CAD build for the part. Positions are in the model's coordinates, mm. Face numbers are marked on the shaded views. A direction names the side the tool comes from. Coordinates: 2 decimals unless noted, no trailing zeros. Order: outer loops, then holes, each group sorted by start corner. A loop starts at its lowest first (then second) coordinate and runs counter-clockwise, first axis right, second up. Notation, with made-up numbers: (42.5, -20.5) - (47.5, -20.5) arc R34 ccw to (47.5, 11.5) - close; hole circle Ø2 at (41, 19). An arc over 180 degrees is marked (long way). Use one line per item in the form item = value.
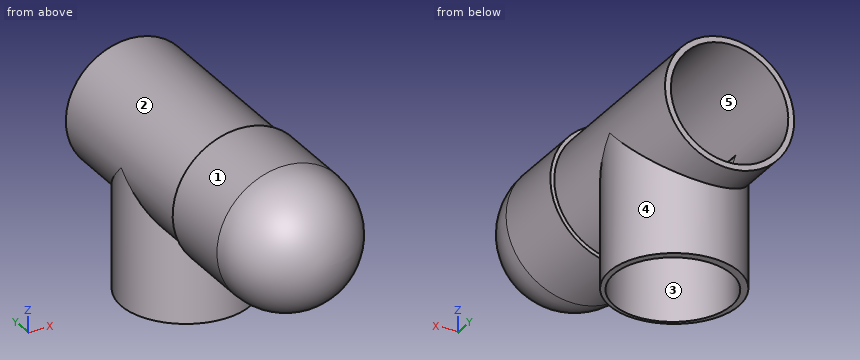
```python
from build123d import *

# Parameters (mm, degrees)
SKETCH1_R                = 15
BOSS_EXTRUDE1_DEPTH      = 70
SKETCH7_R                = 17.5
BOSS_EXTRUDE2_DEPTH      = 20
SKETCH8_R                = 16.5
SKETCH8_R_2              = 15
BOSS_EXTRUDE4_DEPTH      = 70
SKETCH10_R               = 15
CUT_EXTRUDE2_DEPTH       = 70
SKETCH24_R               = 15
CUT_EXTRUDE4_DEPTH       = 22
BOSS_EXTRUDE5_DEPTH      = 15
BOSS_EXTRUDE5_DEPTH_BACK = 20
SKETCH30_R               = 16.5
SKETCH31_R               = 15
CUT_EXTRUDE5_DEPTH       = 37
SKETCH32_R               = 15
CUT_EXTRUDE6_DEPTH       = 55


# Read off the part's stored shape, not the designer's step: Revolve1
with BuildPart() as part:
    # Sketch1 → Boss-Extrude1 (new body)
    with BuildSketch(Plane(origin=(0, 0, 0), x_dir=(1, 0, 0), z_dir=(0, 1, 0))):
        with Locations(Location((0, 0, 0), (0, 0, 270))):
            Circle(SKETCH1_R)
    extrude(amount=-BOSS_EXTRUDE1_DEPTH)

    # Sketch7 → Boss-Extrude2 (add)
    with BuildSketch(Plane.XZ.offset(70)):
        with Locations(Location((0, 0, 0), (0, 0, 270))):
            Circle(SKETCH7_R)
    extrude(amount=-BOSS_EXTRUDE2_DEPTH)

    # Sketch8 → Boss-Extrude4 (add)
    with BuildSketch(Plane(origin=(0, 0, 0), x_dir=(1, 0, 0), z_dir=(0, 1, 0))):
        with Locations(Location((0, 0, 0), (0, 0, 270))):
            Circle(SKETCH8_R)
        Circle(SKETCH8_R_2, mode=Mode.SUBTRACT)
    extrude(amount=-BOSS_EXTRUDE4_DEPTH)

    # Sketch10 → Cut-Extrude2 (cut)
    with BuildSketch(Plane(origin=(0, 0, 0), x_dir=(1, 0, 0), z_dir=(0, 1, 0))):
        with Locations(Location((0, 0, 0), (0, 0, 270))):
            Circle(SKETCH10_R)
    extrude(amount=-CUT_EXTRUDE2_DEPTH, mode=Mode.SUBTRACT)

    # Revolve1 outline → Revolve1 (revolve)
    with BuildSketch(Plane.XY):
        with BuildLine():
            Line((17.5, -69.999999983), (0, -69.999999992))
            Line((0, -69.999999992), (0, -87.5))
            ThreePointArc((0, -87.5), (12.374368677, -82.374368665), (17.5, -69.999999983))
        make_face()
    revolve(axis=Axis((0, 0, 0), (0, 1, 0)))

    # Sketch24 → Cut-Extrude4 (cut)
    with BuildSketch(Plane.XY):
        with Locations((0, -25)):
            Circle(SKETCH24_R)
    extrude(amount=-CUT_EXTRUDE4_DEPTH, mode=Mode.SUBTRACT)

    # Sketch28 → Cut-Revolve1 (revolve, cut)
    with BuildSketch(Plane.XY):
        with BuildLine():
            Line((15, -70), (-15, -70))
            ThreePointArc((-15, -70), (0, -85), (15, -70))
        make_face()
    revolve(axis=Axis((-15, -70, 0), (1, 0, 0)), mode=Mode.SUBTRACT)

    # Sketch30 → Boss-Extrude5 (add, two sides: drawn at the far end of the back side and taken through both)
    with BuildSketch(Plane.XY.offset(-15).offset(-BOSS_EXTRUDE5_DEPTH_BACK)):
        with Locations((0, -25)):
            Circle(SKETCH30_R)
    extrude(amount=BOSS_EXTRUDE5_DEPTH + BOSS_EXTRUDE5_DEPTH_BACK)

    # Sketch31 → Cut-Extrude5 (cut)
    with BuildSketch(Plane(origin=(0, 0, -35), x_dir=(-1, 0, 0), z_dir=(0, 0, -1))):
        with Locations((0, -25.611375347)):
            Circle(SKETCH31_R)
    extrude(amount=-CUT_EXTRUDE5_DEPTH, mode=Mode.SUBTRACT)

    # Sketch32 → Cut-Extrude6 (cut)
    with BuildSketch(Plane(origin=(0, 0, 0), x_dir=(1, 0, 0), z_dir=(0, 1, 0))):
        with Locations(Location((0, 0, 0), (0, 0, 270))):
            Circle(SKETCH32_R)
    extrude(amount=-CUT_EXTRUDE6_DEPTH, mode=Mode.SUBTRACT)


solid = part.part
```
Item 1: Cut at A-A, the plane x = 0. Write the cut outline in (y, z).
Derived:
outline = (-70, -17.5) - (-50, -17.5) - (-50, -16.5) - (-41.5, -16.5) - (-41.5, -35) - (-40.61, -35) - (-40.61, -15) - (-70, -15) arc R15 cw to (-70, 15) - (0, 15) - (0, 16.5) - (-50, 16.5) - (-50, 17.5) - (-70, 17.5) arc R17.5 ccw to start; (-10.61, -35) - (-8.5, -35) - (-8.5, -16.5) - (0, -16.5) - (0, -15) - (-10.61, -15) - close
Item 2: Cut at C-C, the plane z = -1.5. Write the cut outline in (x, y).
Derived:
outline = (-17.44, -70) arc R17.44 ccw to (17.44, -70) - (17.44, -50) - (16.43, -50) - (16.43, -26.5) arc R16.5 ccw to (16.43, -23.5) - (16.43, 0) - (14.92, 0) - (14.92, -24.11) arc R15 cw to (14.92, -27.11) - (14.92, -70) arc R14.92 cw to (-14.92, -70) - (-14.92, -27.11) arc R15 cw to (-14.92, -24.11) - (-14.92, 0) - (-16.43, 0) - (-16.43, -23.5) arc R16.5 ccw to (-16.43, -26.5) - (-16.43, -50) - (-17.44, -50) - close
Item 3: Drop flat-ended pins along their axis: pin 1 (3 mm diameter, centred on y = -44.5, z = -29.5, fed in from -X); pin 2 (5 mm diameter, centred on x = 1, z = -29.5, fed in from +Y); pin 3 (6 mm diameter, centred on x = 0, y = -65, fed in from -Z); pin 4 (5 mm diameter, centred on y = -33, z = -0.5, fed in from -X). Give the stop position or say it passes through.
Derived:
pin_1 = through
pin_2 = -8.5
pin_3 = -17.5
pin_4 = -16.5
Item 4: Two-plate mould, pull along X, no slides. Class the marked faces 3, 4 and 5: +X half, -X half, draft (parallel to the pull), parting line (faces both ways), or undercut.
Derived:
face_3 = undercut
face_4 = parting line
face_5 = undercut
Item 5: Cut at D-D, the plane x = -12. Write the cut outline in (y, z), plus the area to 3 significant figures.
Derived:
outline = (-70, -12.74) - (-50, -12.74) - (-50, -11.32) - (-36.32, -11.32) - (-36.32, -35) - (-34.61, -35) - (-34.61, -9) - (-70, -9) arc R9 cw to (-70, 9) - (0, 9) - (0, 11.32) - (-50, 11.32) - (-50, 12.74) - (-70, 12.74) arc R12.74 ccw to start; (-16.61, -35) - (-13.68, -35) - (-13.68, -11.32) - (0, -11.32) - (0, -9) - (-16.61, -9) - close
area = 578 mm²
Item 6: Cut at B-B, the plane y = -59. Write the cut outline in (x, z).
Derived:
outline = circle Ø35 at (0, 0); hole circle Ø30 at (0, 0)
Item 7: Drill centre lines: line 1 (Z direction, x = 0, y = -54); line 2 (X direction, y = -48, z = 0); line 3 (Y direction, x = 0, z = -23). Where is each one in solid material? Low to high. Write a range as [from, to].
Derived:
line_1 = [-17.5, -15], [15, 17.5]
line_2 = [-16.5, -15], [15, 16.5]
line_3 = [-41.5, -40.61], [-10.61, -8.5]
Item 8: 3-axis set-ups, long thin cutter, end or side, ignore diameter. For the marked faces 1 and 2: which of +Z, -Z, +X, -X, +Y, -Y reach the whole face in a straight line?
Derived:
face_1 = -Y
face_2 = none
